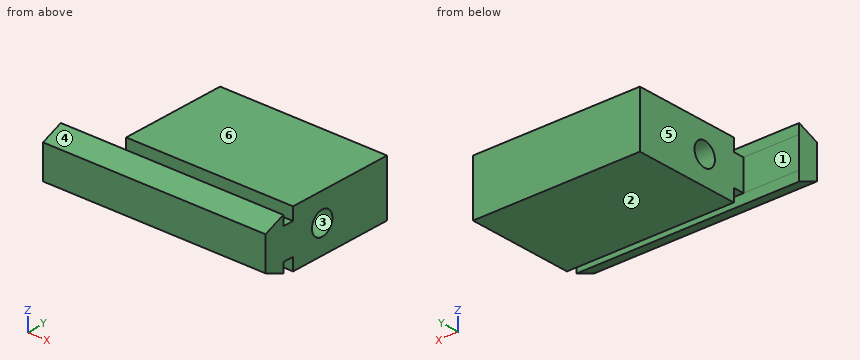
from build123d import *

# Parameters (mm, degrees)
SKETCH_W        = 40
SKETCH_H        = 25
PAD_DEPTH       = 10
POCKET_DEPTH    = 40.001
SKETCH002_R     = 2.1
POCKET001_DEPTH = 40.001
SKETCH003_W     = 21.335087
SKETCH003_H     = 10
POCKET002_DEPTH = 10


with BuildPart() as part:
    # Sketch → Pad (new body)
    with BuildSketch(Plane.XY):
        Rectangle(SKETCH_W, SKETCH_H)
    extrude(amount=-PAD_DEPTH)

    # Sketch001 → Pocket (cut, through all)
    with BuildSketch(Plane.YZ.offset(20)):
        Polygon((-8.835087, -0.5), (-8.835087, -2.25), (-6.835087, -2.25), (-6.835087, 0), (-12.5, 0), (-12.5, -2), align=None)
        Polygon((-8.835087, -9.5), (-8.835087, -7.75), (-6.835087, -7.75), (-6.835087, -10), (-12.5, -10), (-12.5, -8), align=None)
    extrude(amount=-POCKET_DEPTH, mode=Mode.SUBTRACT)

    # Sketch002 (on Face5 of Pocket) → Pocket001 (cut, through all)
    with BuildSketch(Plane(origin=(-20, 0, 0), x_dir=(0, -1, 0), z_dir=(-1, 0, 0))):
        with Locations((0.835087, -5)):
            Circle(SKETCH002_R)
    extrude(amount=-POCKET001_DEPTH, mode=Mode.SUBTRACT)

    # Sketch003 (on Face5 of Pocket001) → Pocket002 (cut)
    with BuildSketch(Plane(origin=(-20, 0, 0), x_dir=(0, -1, 0), z_dir=(-1, 0, 0))):
        with Locations((-1.832457, -5)):
            Rectangle(SKETCH003_W, SKETCH003_H)
    extrude(amount=-POCKET002_DEPTH, mode=Mode.SUBTRACT)


solid = part.part
The listing builds one solid part. Answer for the finished solid, in the listing's coordinates (mm). Face numbers are marked on the shaded views. A direction names the side the tool comes from. Coordinates: 2 decimals unless noted, no trailing zeros. Order: outer loops, then holes, each group sorted by start corner. A loop starts at its lowest first (then second) coordinate and runs counter-clockwise, first axis right, second up.
Q1. A cutting plane is placed at C-C, the plane y = 0.5. Write down the section's boundary in (x, z), and give its area (3 significant figures).
Q2. Consider line 1 (Y direction, x = 4, z = -6); line 2 (Y direction, x = -18, z = -5.25); line 3 (X direction, y = -0.25, z = -7.5). Determine where each line is inside the solid, lowest interval first.
Q3. A cutting plane is placed at A-A, the plane x = 16. Write down the section's boundary in (y, z).
Q4. A cutting plane is placed at D-D, the plane y = 3.75. Write down the section's boundary in (x, z).
Q5. For a pull along Y with two mould halves and no side action, classify the marked faces 1, 2, 3 and 4 as pulls with the +Y half, pulls with the -Y half, needs draft (parallel to the pull), parting line crosses it, or undercut.
Q6. Which of the six approach directions +Z, -Z, +X, -X, +Y, -Y give full straight-line access (tool end or side, diameter ignored) to the marked faces 5 and 6?
Q7. Given P1, Ø2, axis at y = 9, z = -7, coming from the -X side; P2, Ø0.7, axis at x = 9, z = -0.5, coming from the -Y side; P3, Ø1, axis at x = 3, y = -8, coming from the +Z side; P4, Ø3.5, axis at y = -0.84, z = -5, coming from the +X side, each flat-ended and moving along its own axis, determine where each tip first touches the part or whether it passes through.
Q8. A cutting plane is placed at B-B, the plane z = -5. Write down the section's boundary in (x, y).
Answers follow:
1. outline: (-10, -10) - (20, -10) - (20, -6.62) - (-10, -6.62) - close; (-10, -3.38) - (20, -3.38) - (20, 0) - (-10, 0) - close
1. area: 203 mm2
2. line 1: y = -12.5 to -2.68, 1.01 to 12.5
2. line 2: y = -12.5 to -8.84
2. line 3: x = -10 to 20
3. outline: (-12.5, -8) - (-8.84, -9.5) - (-8.84, -7.75) - (-6.84, -7.75) - (-6.84, -10) - (12.5, -10) - (12.5, 0) - (-6.84, 0) - (-6.84, -2.25) - (-8.84, -2.25) - (-8.84, -0.5) - (-12.5, -2) - close; hole circle Ø4.2 at (-0.84, -5)
4. outline: (-10, -10) - (20, -10) - (20, 0) - (-10, 0) - close
5. face 1: pulls with the +Y half
5. face 2: needs draft
5. face 3: undercut
5. face 4: pulls with the -Y half
6. face 5: +Z, -Z, -X, +Y
6. face 6: +Z, +X, -X, +Y, -Y
7. P1: stops at x = -10
7. P2: stops at y = -9.69
7. P3: stops at z = -2.25
7. P4: passes through
8. outline: (-20, -12.5) - (20, -12.5) - (20, -2.94) - (-10, -2.94) - (-10, -8.84) - (-20, -8.84) - close; (-10, 1.26) - (20, 1.26) - (20, 12.5) - (-10, 12.5) - close
